Part model, mm, in its own coordinate system. A direction names the side the tool comes from. Coordinates: 2 decimals unless noted, no trailing zeros. Loops run counter-clockwise (first coordinate to the right, second up) from the corner with the lowest first, then second, coordinate; pieces in that order, holes last. Notation, with made-up numbers: (-32.5, 49) - (20.5, 49) arc R17 ccw to (20.5, 54) - close; hole circle Ø11 at (-10, 65.25). An arc over 180 degrees is marked (long way). Use a Markdown table: item, result. Add a question column.
1. Band-saw the part on A-A, the plane x = 4.75. Give the cut face in (y, z).
2. Drop flat-ended pins along their axis: pin 1 (0.8 mm diameter, centred on x = 0, y = 3, fed in from -Z); pin 2 (0.8 mm diameter, centred on y = 2.5, z = 0, fed in from +X). Give the stop position or say it passes through.
3. Band-saw the part on D-D, the plane y = 0.5. Give the cut face in (x, z), plus the area to 3 significant figures.
4. Band-saw the part on B-B, the plane y = 2.8. Give the cut face in (x, z).
5. Wall check: probe 1 along X at (y, z) = (2.05, 1.75); probe 2 along Z at (x, y) = (0.25, 3.3); probe 3 along Z at (x, y) = (-4.75, 0.95). Give the ranges that are in metal, low to high. Write a range as [from, to].
6. 3-axis set-ups, long thin cutter, end or side, ignore diameter. For faces 4 (the cylindrical face through (6.715, 2.76, -4.449)), 5 (the flat face through (0, 3, 4.75)), 6 (the flat face through (7, 3, 0)), 7 (the cylindrical face through (-6.699, 2.76, 4.465)), 8 (the flat face through (-7, 3, 0)): which of +Z, -Z, +X, -X, +Y, -Y reach the whole face in a straight line?
7. Band-saw the part on C-C, the plane z = 1.75. Give the cut face in (x, y), plus the area to 3 significant figures.
8. Pull direction Y, two halves, no side cores. Call faces 1 (the cylindrical face through (0.098, 0.301, 5.465)), 2 (the flat face through (0, 2, -5)), 3 (the cylindrical face through (-6.699, 2.76, -4.465)): pulls with the +Y half, pulls with the -Y half, needs draft (parallel to the pull), parting line crosses it, or undercut.
from build123d import *

# Parameters (mm, degrees)
CROQUIS1_W              = 16
CROQUIS1_H              = 11.5
SALIENTE_EXTRUIR2_DEPTH = 2
CROQUIS2_W              = 14
CROQUIS2_H              = 9.5
SALIENTE_EXTRUIR3_DEPTH = 2
REDONDEO1_R             = 1
REDONDEO2_R             = 1
REDONDEO3_R             = 0.5


with BuildPart() as part:
    # Croquis1 → Saliente-Extruir2 (new body)
    with BuildSketch(Plane(origin=(0, 0, 0), x_dir=(1, 0, 0), z_dir=(0, 1, 0))):
        Rectangle(CROQUIS1_W, CROQUIS1_H)
    extrude(amount=SALIENTE_EXTRUIR2_DEPTH)

    # Croquis2 → Saliente-Extruir3 (add)
    with BuildSketch(Plane(origin=(0, 2, 0), x_dir=(1, 0, 0), z_dir=(0, 1, 0))):
        Rectangle(CROQUIS2_W, CROQUIS2_H)
    extrude(amount=SALIENTE_EXTRUIR3_DEPTH)

    # Redondeo1
    redondeo1_edges = [part.edges().sort_by_distance(p)[0] for p in [
        (0, 0, 5.75),
        (8, 0, 0),
        (0, 0, -5.75),
        (-8, 0, 0),
        (-8, 1, 5.75),
        (8, 1, 5.75),
        (8, 1, -5.75),
        (-8, 1, -5.75),
    ]]
    fillet(redondeo1_edges, radius=REDONDEO1_R)

    # Redondeo2
    redondeo2_edges = [part.edges().sort_by_distance(p)[0] for p in [
        (7, 3, 4.75),
        (7, 3, -4.75),
        (-7, 3, -4.75),
        (-7, 3, 4.75),
    ]]
    fillet(redondeo2_edges, radius=REDONDEO2_R)

    # Redondeo3
    redondeo3_edges = [part.edges().sort_by_distance(p)[0] for p in [
        (7, 4, 0),
        (0, 4, 4.75),
        (0, 4, -4.75),
        (-7, 4, 0),
        (-6.707106781, 4, 4.457106781),
        (-6.707106781, 4, -4.457106781),
        (6.707106781, 4, -4.457106781),
        (6.707106781, 4, 4.457106781),
    ]]
    fillet(redondeo3_edges, radius=REDONDEO3_R)


solid = part.part
Geometry check:
| question | item | result |
|---|---|---|
| 1 | outline | (0, -4.75) arc R1 ccw to (1, -5.75) - (2, -5.75) - (2, -4.75) - (3.5, -4.75) arc R0.5 ccw to (4, -4.25) - (4, 4.25) arc R0.5 ccw to (3.5, 4.75) - (2, 4.75) - (2, 5.75) - (1, 5.75) arc R1 ccw to (0, 4.75) - close |
| 2 | pin 1 | stops at z = -4.75 |
| 2 | pin 2 | stops at x = 7 |
| 3 | outline | (-7.87, -4.75) arc R0.87 ccw to (-7, -5.62) - (7, -5.62) arc R0.87 ccw to (7.87, -4.75) - (7.87, 4.75) arc R0.87 ccw to (7, 5.62) - (-7, 5.62) arc R0.87 ccw to (-7.87, 4.75) - close |
| 3 | area | 176 mm^2 |
| 4 | outline | (-7, -3.75) arc R1 ccw to (-6, -4.75) - (6, -4.75) arc R1 ccw to (7, -3.75) - (7, 3.75) arc R1 ccw to (6, 4.75) - (-6, 4.75) arc R1 ccw to (-7, 3.75) - close |
| 5 | probe 1 | x = [-7, 7] |
| 5 | probe 2 | z = [-4.75, 4.75] |
| 5 | probe 3 | z = [-5.75, 5.75] |
| 6 | face 4 | -Z, +X, +Y |
| 6 | face 5 | +Z, +X, -X, +Y |
| 6 | face 6 | +Z, -Z, +X, +Y |
| 6 | face 7 | +Z, -X, +Y |
| 6 | face 8 | +Z, -Z, -X, +Y |
| 7 | outline | (-8, 1) arc R1 ccw to (-7, 0) - (7, 0) arc R1 ccw to (8, 1) - (8, 2) - (7, 2) - (7, 3.5) arc R0.5 ccw to (6.5, 4) - (-6.5, 4) arc R0.5 ccw to (-7, 3.5) - (-7, 2) - (-8, 2) - close |
| 7 | area | 59.5 mm^2 |
| 8 | face 1 | pulls with the -Y half |
| 8 | face 2 | pulls with the +Y half |
| 8 | face 3 | needs draft |
